Here's how the part is built. I have some questions about the finished solid (model axes, mm). A direction names the side the tool comes from. Coordinates: 2 decimals unless noted, no trailing zeros. Order: outer loops, then holes, each group sorted by start corner. A loop starts at its lowest first (then second) coordinate and runs counter-clockwise, first axis right, second up. Notation, with made-up numbers: (22, 8.25) - (40, 8.25) arc R21 cw to (40, 20.25) - close; hole circle Ø11 at (-10.75, 30). An arc over 180 degrees is marked (long way). Answer as CSV lines item,"result". Start each with the question number.
Q1. Suppose I cut it at B-B (x = -5.5). Please give me the cut outline in (y, z).
Q2. For faces 1 (the face through (0, 18, 17.5)), 2 (the face through (-1, 0, 0)), which set-ups out of +Z, -Z, +X, -X, +Y, -Y let a thin tool reach every point of the face, with its end or its side?
Q3. I need wall thicknesses on line 1 (X direction, y = 16.5, z = 6); line 2 (Z direction, x = 18.5, y = 18.75); line 3 (Y direction, x = 24, z = 0). Which ranges of each line are inside material? Lowest first, please.
Q4. For pin 1 Ø2 at (x, z) = (31.5, 4.5) entering from -Y; pin 2 Ø2 at (x, z) = (-30, 9.5) entering from +Y, each with a flat end and sliding along its axis, tell me the tip position at first contact or that it passes through.
Q5. Suppose I cut it at A-A (z = -2). Please give me the cut outline in (x, y), then the cut area to 3 significant figures.
Q6. Suppose I cut it at C-C (z = 20.5). Please give me the cut outline in (x, y).
Q7. Thinking about a two-plate mould opening in Z: for faces 3 (the face through (-1, 10, 25)), 4 (the face through (-36.99, 17.46, 14.65)), 5 (the face through (-1, 20, -23)), 6 (the face through (-1, 10, -25)), which applies, released by +Z, released by -Z, zero draft, split by the parting line, or undercut?
Q8. Suppose I cut it at D-D (z = -22). Please give me the cut outline in (x, y).
from build123d import *

# Parameters (mm, degrees)
SKETCH1_W           = 100
SKETCH1_H           = 50
BOSS_EXTRUDE1_DEPTH = 20
SKETCH2_W           = 80
SKETCH2_H           = 35
CUT_EXTRUDE1_DEPTH  = 5
FILLET1_R           = 10
FILLET2_R           = 10


with BuildPart() as part:
    # Sketch1 → Boss-Extrude1 (new body)
    with BuildSketch(Plane(origin=(0, 0, 0), x_dir=(1, 0, 0), z_dir=(0, 1, 0))):
        Rectangle(SKETCH1_W, SKETCH1_H)
    extrude(amount=BOSS_EXTRUDE1_DEPTH)

    # Sketch2 → Cut-Extrude1 (cut)
    with BuildSketch(Plane(origin=(0, 20, 0), x_dir=(1, 0, 0), z_dir=(0, 1, 0))):
        Rectangle(SKETCH2_W, SKETCH2_H)
    extrude(amount=-CUT_EXTRUDE1_DEPTH, mode=Mode.SUBTRACT)

    # Fillet1
    fillet1_edges = [part.edges().sort_by_distance(p)[0] for p in [
        (-50, 10, -25),
        (50, 10, -25),
        (50, 10, 25),
        (-50, 10, 25),
    ]]
    fillet(fillet1_edges, radius=FILLET1_R)

    # Fillet2
    fillet2_edges = [part.edges().sort_by_distance(p)[0] for p in [
        (-40, 17.5, 17.5),
        (-40, 17.5, -17.5),
        (40, 17.5, -17.5),
        (40, 17.5, 17.5),
    ]]
    fillet(fillet2_edges, radius=FILLET2_R)


solid = part.part
Here are the results:
1,outline,"(0, -25) - (20, -25) - (20, -17.5) - (15, -17.5) - (15, 17.5) - (20, 17.5) - (20, 25) - (0, 25) - close"
2,face 1,"+Y"
2,face 2,"+Z, -Z, +X, -X, -Y"
3,line 1,"x = -50 to -40, 40 to 50"
3,line 2,"z = -25 to -17.5, 17.5 to 25"
3,line 3,"y = 0 to 15"
4,pin 1,"stops at y = 0"
4,pin 2,"stops at y = 15"
5,outline,"(-50, 0) - (50, 0) - (50, 20) - (40, 20) - (40, 15) - (-40, 15) - (-40, 20) - (-50, 20) - close"
5,area,"1,600 mm²"
6,outline,"(-48.35, 0) - (48.35, 0) - (48.35, 20) - (-48.35, 20) - close"
7,face 3,"released by +Z"
7,face 4,"undercut"
7,face 5,"zero draft"
7,face 6,"released by -Z"
8,outline,"(-47.14, 0) - (47.14, 0) - (47.14, 20) - (-47.14, 20) - close"
